Verification items for this drawing (mm, ordinates from the low corner). Give positions to 0.01 mm unless a question says otherwise; leave off trailing zeros. Loops run counter-clockwise (first coordinate to the right, second up) from the corner with the lowest first, then second, coordinate; pieces in that order, holes last. Notation, with made-up numbers: (-32, 18.25) -> (-9, 18.25) arc R13 ccw to (-9, 30.25) -> close; hole circle Ø6 at (-13.75, -23.75). An arc over 180 degrees is marked (long way). Answer in a Markdown table with one row per item. Add a question column.
Q1. Section check A-A on y = 14.5. Enter the section's corners in (x, z).
Q2. Section check C-C on z = 0.2. Enter the section's corners in (x, y), and give its area (3 significant figures).
Q3. Section check B-B on x = 6.5. Enter the section's corners in (y, z).
Q4. Material ranges on probe 1 along X at (y, z) = (19, 0.65) (1 decimal); probe 2 along Y at (x, z) = (12, 0.2); probe 3 along X at (y, z) = (29, 0.55) (1 decimal), recorded low to high.
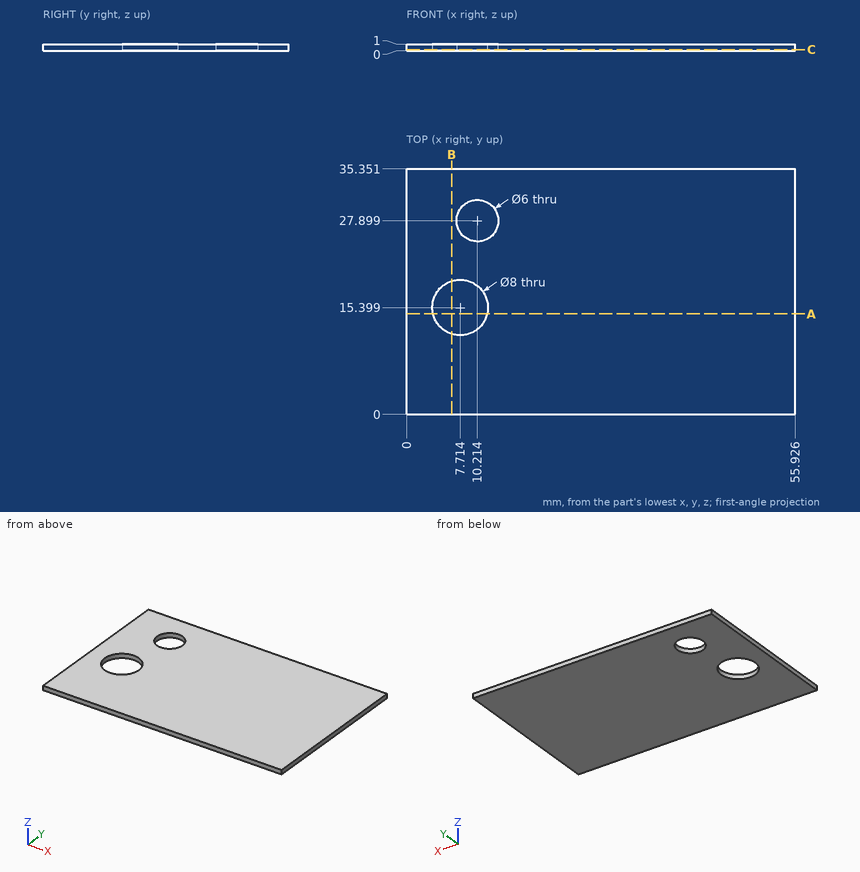
Taken from the geometry:
| question | item | result |
|---|---|---|
| 1 | outline | (0, 0) -> (3.82, 0) -> (3.82, 1) -> (0, 1) -> close; (11.61, 0) -> (55.93, 0) -> (55.93, 1) -> (11.61, 1) -> close |
| 2 | outline | (0, 0) -> (55.93, 0) -> (55.93, 35.35) -> (0, 35.35) -> close; hole circle Ø8 at (7.71, 15.4); hole circle Ø6 at (10.21, 27.9) |
| 2 | area | 1,900 mm² |
| 3 | outline | (0, 0) -> (11.59, 0) -> (11.59, 1) -> (0, 1) -> close; (19.21, 0) -> (35.35, 0) -> (35.35, 1) -> (19.21, 1) -> close |
| 4 | probe 1 | x = 0 to 6, 9.5 to 55.9 |
| 4 | probe 2 | y = 0 to 25.49, 30.31 to 35.35 |
| 4 | probe 3 | x = 0 to 7.4, 13 to 55.9 |
